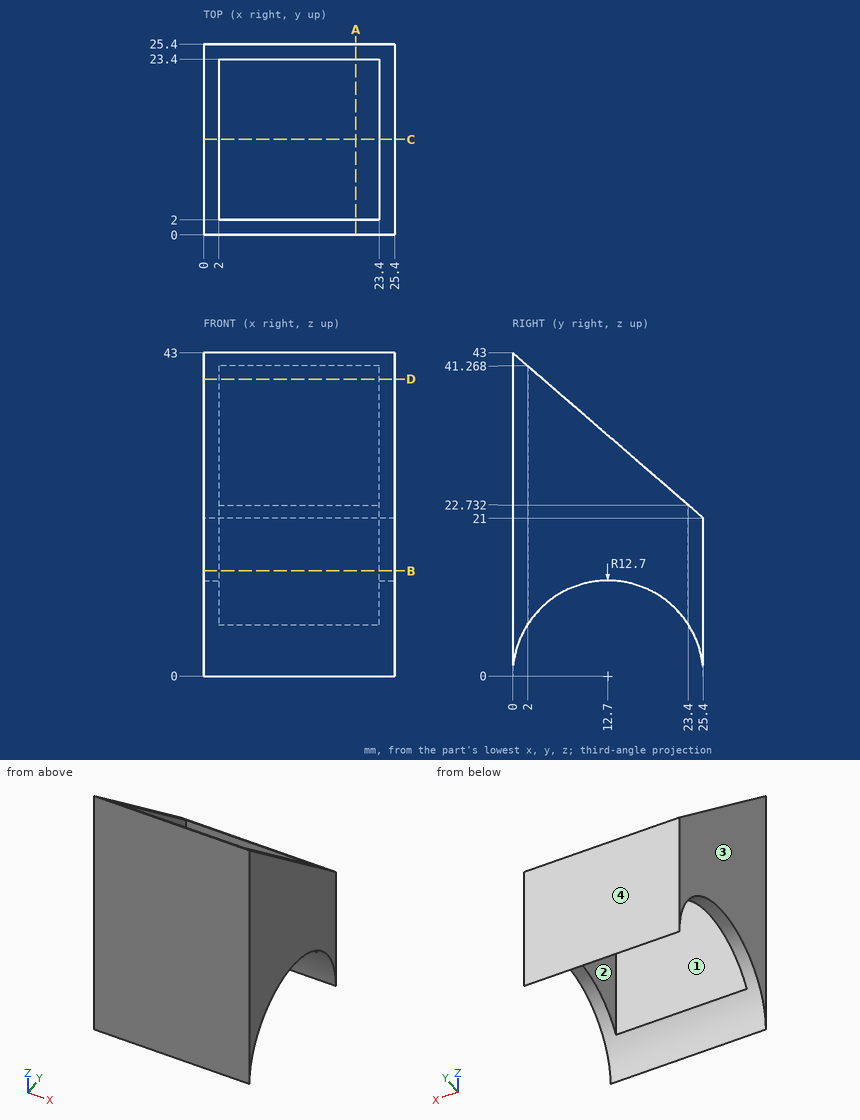
Design review of the part shown in the three views and the two pictorial views. Dimensions are in mm from the part's minimum x, y and z. Coordinates: 2 decimals unless noted, no trailing zeros. Loops run counter-clockwise (first coordinate to the right, second up) from the corner with the lowest first, then second, coordinate; pieces in that order, holes last. Notation, with made-up numbers: M 73,54 L 116,54 A29 cw 116,79 Z; hole C 15.25,26.25 d8. An arc over 180 degrees is marked long. One line per question, with ' | ' between items.
(1) For pin 1 Ø6 at (x, y) = (4, 7) entering from -Z (1 decimal), flat-tipped, find the tip position at first contact; note if it passes through.
Filled in:
pin 1: stops at z = 9.9
(2) We need section D-D (z = 39.5). Give the boundary of the cut face in (x, y).
Filled in:
outline: M 0,0 L 25.4,0 L 25.4,4.04 L 23.4,4.04 L 23.4,2 L 2,2 L 2,4.04 L 0,4.04 Z
(3) Wall thickness on probe 1 along X at (y, z) = (17.5, 19); probe 2 along Y at (x, z) = (14.5, 35.5): over which ranges is each line inside the solid? List them lowest first.
Filled in:
probe 1: x = 0 to 2, 23.4 to 25.4 | probe 2: y = 0 to 2
(4) We need section A-A (x = 20.25). Give the boundary of the cut face in (y, z).
Filled in:
outline: M 0,0 A12.7 cw 2,6.84 L 2,41.27 L 0,43 Z; M 23.4,6.84 A12.7 cw 25.4,0 L 25.4,21 L 23.4,22.73 Z
(5) We need section B-B (z = 14). Give the boundary of the cut face in (x, y), and give its area (3 significant figures).
Filled in:
outline: M 0,0 L 25.4,0 L 25.4,25.4 L 0,25.4 Z; hole M 2,2 L 23.4,2 L 23.4,23.4 L 2,23.4 Z | area: 187 mm^2
(6) We need section C-C (y = 12.7). Give the boundary of the cut face in (x, z).
Filled in:
outline: M 0,12.7 L 2,12.7 L 2,32 L 0,32 Z; M 23.4,12.7 L 25.4,12.7 L 25.4,32 L 23.4,32 Z
(7) Draft analysis for pull direction X (two halves, no side actions). For the marked faces 1, 2, 3 and 4, state which applies: released by +X, released by -X, zero draft, split by the parting line, or undercut.
Filled in:
face 1: undercut | face 2: undercut | face 3: released by -X | face 4: zero draft
